```python
from build123d import *

# Parameters (mm, degrees)
SKETCH1_W                = 133.2
SKETCH1_H                = 133.2
SKETCH1_W_2              = 127.2
SKETCH1_H_2              = 127.2
BOSS_EXTRUDE1_DEPTH      = 50
SKETCH2_W                = 127.2
SKETCH2_H                = 127.2
BOSS_EXTRUDE2_DEPTH      = 3
BOSS_EXTRUDE4_DEPTH      = 7
BOSS_EXTRUDE4_DEPTH_BACK = 3
SKETCH3_R                = 3.625
SKETCH4_W                = 127.2
SKETCH4_H                = 30
CUT_EXTRUDE2_DEPTH       = 158.091692969
CUT_EXTRUDE3_DEPTH       = 158.091692969
CUT_EXTRUDE6_DEPTH       = 106.262148943


with BuildPart() as part:
    # Sketch1 → Boss-Extrude1 (new body)
    with BuildSketch(Plane(origin=(0, 0, 0), x_dir=(1, 0, 0), z_dir=(0, 1, 0))):
        Rectangle(SKETCH1_W, SKETCH1_H)
        Rectangle(SKETCH1_W_2, SKETCH1_H_2, mode=Mode.SUBTRACT)
    extrude(amount=BOSS_EXTRUDE1_DEPTH)

    # Sketch2 → Boss-Extrude2 (add)
    with BuildSketch(Plane(origin=(0, 0, 0), x_dir=(1, 0, 0), z_dir=(0, 1, 0))):
        Rectangle(SKETCH2_W, SKETCH2_H)
    extrude(amount=BOSS_EXTRUDE2_DEPTH)

    # Sketch3 → Boss-Extrude4 (add, two sides: drawn at the far end of the back side and taken through both)
    # profile 1 of 4: a face of its own
    with BuildSketch(Plane(origin=(0, 3, 0), x_dir=(1, 0, 0), z_dir=(0, 1, 0)).offset(-BOSS_EXTRUDE4_DEPTH_BACK)):
        with BuildLine():
            ThreePointArc((-63.6, 51.6), (-55.371805983, 55.371805983), (-51.6, 63.6))
            Line((-51.6, 63.6), (-63.6, 63.6))
            Line((-63.6, 63.6), (-63.6, 51.6))
        make_face()
        with Locations(Location((-58.6, 58.6, 0), (0, 0, 270))):
            Circle(SKETCH3_R, mode=Mode.SUBTRACT)
    # profile 2 of 4: a face of its own
    with BuildSketch(Plane(origin=(0, 3, 0), x_dir=(1, 0, 0), z_dir=(0, 1, 0)).offset(-BOSS_EXTRUDE4_DEPTH_BACK)):
        with BuildLine():
            ThreePointArc((-51.902705138, -63.6), (-55.559775075, -55.463705987), (-63.6, -51.6))
            Line((-63.6, -51.6), (-63.6, -63.6))
            Line((-63.6, -63.6), (-51.902705138, -63.6))
        make_face()
        with Locations(Location((-58.6, -58.6, 0), (0, 0, 90))):
            Circle(SKETCH3_R, mode=Mode.SUBTRACT)
    # profile 3 of 4: a face of its own
    with BuildSketch(Plane(origin=(0, 3, 0), x_dir=(1, 0, 0), z_dir=(0, 1, 0)).offset(-BOSS_EXTRUDE4_DEPTH_BACK)):
        with BuildLine():
            Line((63.6, 63.6), (51.6, 63.6))
            ThreePointArc((51.6, 63.6), (55.375031477, 55.378323531), (63.6, 51.610470108))
            Line((63.6, 51.610470108), (63.6, 63.6))
        make_face()
        with Locations(Location((58.6, 58.6, 0), (0, 0, 90))):
            Circle(SKETCH3_R, mode=Mode.SUBTRACT)
    # profile 4 of 4: a face of its own
    with BuildSketch(Plane(origin=(0, 3, 0), x_dir=(1, 0, 0), z_dir=(0, 1, 0)).offset(-BOSS_EXTRUDE4_DEPTH_BACK)):
        with BuildLine():
            Line((63.6, -63.6), (63.6, -51.6))
            ThreePointArc((63.6, -51.6), (55.371805983, -55.371805983), (51.6, -63.6))
            Line((51.6, -63.6), (63.6, -63.6))
        make_face()
        with Locations(Location((58.6, -58.6, 0), (0, 0, 270))):
            Circle(SKETCH3_R, mode=Mode.SUBTRACT)
    extrude(amount=BOSS_EXTRUDE4_DEPTH + BOSS_EXTRUDE4_DEPTH_BACK)

    # Sketch4 → Cut-Extrude2 (cut, through all)
    with BuildSketch(Plane(origin=(66.6, 0, 0), x_dir=(0, 0, -1), z_dir=(1, 0, 0))):
        with Locations((0, 24.5)):
            Rectangle(SKETCH4_W, SKETCH4_H)
    extrude(amount=-CUT_EXTRUDE2_DEPTH, mode=Mode.SUBTRACT)

    # Sketch5 → Cut-Extrude3 (cut, through all)
    with BuildSketch(Plane(origin=(66.6, 0, 0), x_dir=(0, 0, -1), z_dir=(1, 0, 0))):
        Polygon((-50, 48.25), (-50, 46.5), (50, 46.5), (50, 48.25), (48, 48.25), (47, 49.25), (47, 50), (-47, 50), (-47, 49.25), (-48, 48.25), align=None)
    extrude(amount=-CUT_EXTRUDE3_DEPTH, mode=Mode.SUBTRACT)

    # Sketch6 → Cut-Extrude6 (cut, through all)
    with BuildSketch(Plane(origin=(0, 3, 0), x_dir=(1, 0, 0), z_dir=(0, 1, 0))):
        Polygon((-53.053423166, -55.371805983), (-55.371805983, -55.371805983), (-55.371805983, -50), (-5.371805983, 0), (50, 55.371805983), (55.371805983, 55.371805983), (55.371805983, 53.053423166), (53.8450944, 51.526711583), (-1.526711583, -3.8450944), (-5.371805983, -7.690188801), align=None)
        Polygon((-55.371805983, -37.690188801), (-55.371805983, -30), (-25.371805983, 0), (30, 55.371805983), (37.690188801, 55.371805983), (33.8450944, 51.526711583), (-21.526711583, -3.8450944), (-25.371805983, -7.690188801), align=None)
        Polygon((-55.371805983, -27.690188801), (-55.371805983, -20), (-35.371805983, 0), (20, 55.371805983), (27.690188801, 55.371805983), (23.8450944, 51.526711583), (-31.526711583, -3.8450944), (-35.371805983, -7.690188801), align=None)
        Polygon((-55.371805983, -17.690188801), (-55.371805983, -10), (-45.371805983, 0), (10, 55.371805983), (17.690188801, 55.371805983), (13.8450944, 51.526711583), (-41.526711583, -3.8450944), (-45.371805983, -7.690188801), align=None)
        Polygon((0, 55.371805983), (7.690188801, 55.371805983), (3.8450944, 51.526711583), (-51.526711583, -3.8450944), (-55.371805983, -7.690188801), (-55.371805983, 0), align=None)
        with BuildLine():
            ThreePointArc((18.836860938, -37.694136454), (28.265498696, -41.599606087), (37.694136454, -37.694136454))
            Line((37.694136454, -37.694136454), (28.265498696, -28.265498696))
            Line((28.265498696, -28.265498696), (18.836860938, -37.694136454))
        make_face()
        with BuildLine():
            Line((41.229670359, -15.301327032), (44.765204265, -11.765793127))
            ThreePointArc((44.765204265, -11.765793127), (28.265498696, -4.931391304), (11.765793127, -11.765793127))
            Line((11.765793127, -11.765793127), (15.301327032, -15.301327032))
            Line((15.301327032, -15.301327032), (18.836860938, -18.836860938))
            ThreePointArc((18.836860938, -18.836860938), (28.265498696, -14.931391304), (37.694136454, -18.836860938))
            Line((37.694136454, -18.836860938), (41.229670359, -15.301327032))
        make_face()
        Polygon((-15.371805983, 0), (-55.371805983, -40), (-55.371805983, -47.690188801), (-15.371805983, -7.690188801), (-11.526711583, -3.8450944), (43.8450944, 51.526711583), (47.690188801, 55.371805983), (40, 55.371805983), align=None)
    extrude(amount=-CUT_EXTRUDE6_DEPTH, mode=Mode.SUBTRACT)


solid = part.part
```
Could you check a few things on this model? Use its own coordinates, in mm. A direction names the side the tool comes from. Coordinates: 2 decimals unless noted, no trailing zeros. Write each loop counter-clockwise with the first axis right and the second up, starting at its lowest first coordinate (ties: lowest second). Pieces come first, ordered by that corner, then holes. Notation, with made-up numbers: M 31.25,70 L 64.25,70 A23 ccw 64.25,89 Z; hole C 58.5,30.25 d10. An arc over 180 degrees is marked long. Answer as CSV lines item,"result". Start each with the question number.
1) For faces 4 (the flat face through (-1, 25, -66.6)), 5 (the flat face through (59, 3, -59)), 6 (the flat face through (-65, 39.5, 1)), 7 (the flat face through (15, 2, 15)), which set-ups out of +Z, -Z, +X, -X, +Y, -Y let a thin tool reach every point of the face, with its end or its side?
2) Please list where these lines run through material, in increasing order: line 1 (Z direction, x = 11.5, y = 20.5); line 2 (Z direction, x = -58, y = 7) (3 decimals); line 3 (X direction, y = 6, z = -58) (3 decimals). Write a range as from..to.
3) For P1, Ø2, axis at x = 30.5, z = 44, coming from the +Y side; P2, Ø8.5, axis at x = -58.6, z = 58.6, coming from the -Y side; P3, Ø1.5, axis at x = -65.5, z = 4, coming from the +Y side; P4, Ø8, axis at x = -57, z = 58, coming from the +Y side, each with a flat end and sliding along its axis, tell me the tip position at first contact or that it passes through.
4) I want a section at C-C, the plane z = 58.6. Please give me the cut outline in (x, y) (3 decimals), and give its area (3 significant figures).
5) We'd pull the mould along Z, two halves only. Please class faces 1 (the flat face through (-55.372, 2, 14)), 2 (the flat face through (-1, 25, 66.6)), 3 (the flat face through (66.6, 8, 5)): +Z half, -Z half, draft (parallel to the pull), parting line (faces both ways), or undercut.
6) I want a section at B-B, the plane y = 24. Please give me the cut outline in (x, z).
7) I want a section at D-D, the plane x = -7. Give the number of separate pieces and of enclosed holes in the cut face, and give its area (3 significant figures).
8) I want a section at A-A, the plane y = 7. Please give me the cut outline in (x, z) (3 decimals).
Data:
1,face 4,"-Z, +X, -X, +Y, -Y"
1,face 5,"+Y"
1,face 6,"+X, -X"
1,face 7,"+Y, -Y"
2,line 1,"z = -66.6..-63.6, 63.6..66.6"
2,line 2,"z = -66.6..-62.175, -55.025..-53.343, 53.501..55.025, 62.175..66.6"
2,line 3,"x = -66.6..-62.175, -55.025..-53.343, 53.349..55.025, 62.175..66.6"
3,P1,"stops at y = 3"
3,P2,"stops at y = 0"
3,P3,"stops at y = 46.5"
3,P4,"stops at y = 9.5"
4,outline,"M -66.6,0 L 66.6,0 L 66.6,9.5 L 62.225,9.5 L 62.225,3 L 54.975,3 L 54.975,9.5 L 53.013,9.5 L 53.013,3 L -53.304,3 L -53.304,9.5 L -54.975,9.5 L -54.975,3 L -62.225,3 L -62.225,9.5 L -66.6,9.5 Z; M -66.6,39.5 L -63.6,39.5 L -63.6,50 L -66.6,50 Z; M 63.6,39.5 L 66.6,39.5 L 66.6,50 L 63.6,50 Z"
4,area,"543 mm^2"
5,face 1,"undercut"
5,face 2,"+Z half"
5,face 3,"draft"
6,outline,"M -66.6,-66.6 L 66.6,-66.6 L 66.6,-63.6 L -66.6,-63.6 Z; M -66.6,63.6 L 66.6,63.6 L 66.6,66.6 L -66.6,66.6 Z"
7,separate pieces,"7"
7,enclosed holes,"0"
7,area,"543 mm^2"
8,outline,"M -66.6,-66.6 L 66.6,-66.6 L 66.6,66.6 L -66.6,66.6 Z; hole M -63.6,-51.6 A13 cw -51.6,-63.6 L 51.6,-63.6 A13 cw 63.6,-51.61 L 63.6,51.6 A13 cw 51.6,63.6 L -51.903,63.6 A13 cw -63.6,51.6 Z; hole C -58.6,-58.6 d7.25; hole C -58.6,58.6 d7.25; hole C 58.6,-58.6 d7.25; hole C 58.6,58.6 d7.25"
